Source: CAD feature listing. Evaluate the final solid. Frame: model axes, mm. A direction names the side the tool comes from. Give positions to 0.01 mm unless a question says otherwise; leave off trailing zeros. Loops run counter-clockwise (first coordinate to the right, second up) from the corner with the lowest first, then second, coordinate; pieces in that order, holes last.
```python
from build123d import *

# Parameters (mm, degrees)
SKETCH_1_W          = 16.2
SKETCH_1_H          = 16.9
EXTRUDE_1_DEPTH     = 16.9
CUT_EXTRUDE_1_DEPTH = 10
SKETCH_3_W          = 2.946300562
SKETCH_3_H          = 2.060350043
CUT_EXTRUDE_2_DEPTH = 0.2
SKETCH_4_W          = 14.323300114
SKETCH_4_H          = 2.725353119
CUT_EXTRUDE_3_DEPTH = 0.1
SKETCH_5_W          = 12.529891582
SKETCH_5_H          = 0.500524342
CUT_EXTRUDE_4_DEPTH = 0.1
CHAMFER_1_SIZE      = 0.5
CUT_EXTRUDE_5_DEPTH = 0.1
FILLET_1_R          = 0.1
SKETCH_7_R          = 1.25
SKETCH_7_W          = 0.5
SKETCH_7_H          = 0.4
SKETCH_7_H_2        = 0.5
SKETCH_7_W_2        = 0.3
SKETCH_7_H_3        = 1.2
EXTRUDE_2_DEPTH     = 3.3


with BuildPart() as part:
    # Эскиз1 → Бобышка-Вытянуть1 (new body)
    with BuildSketch(Plane.XY):
        Rectangle(SKETCH_1_W, SKETCH_1_H)
    extrude(amount=EXTRUDE_1_DEPTH)

    # Эскиз2 → Вырез-Вытянуть1 (cut)
    with BuildSketch(Plane.XY.offset(16.9)):
        Polygon((-6.264945791, -3.803921673), (-6.264945791, 4.664369649), (-3.10783524, 4.664369649), (-3.10783524, 6.730894781), (-1.828998264, 6.730894781), (-1.828998264, 7.89024711), (1.828998264, 7.89024711), (1.828998264, 6.730894781), (3.10783524, 6.730894781), (3.10783524, 4.664369649), (6.264945791, 4.664369649), (6.264945791, -3.803921673), align=None)
    extrude(amount=-CUT_EXTRUDE_1_DEPTH, mode=Mode.SUBTRACT)

    # Эскиз3 → Вырез-Вытянуть2 (cut)
    with BuildSketch(Plane.XY.offset(16.9)):
        with Locations((-5.415203287, 6.790232272)):
            Rectangle(SKETCH_3_W, SKETCH_3_H)
        with Locations((5.415203287, 6.790232272)):
            Rectangle(SKETCH_3_W, SKETCH_3_H)
    extrude(amount=-CUT_EXTRUDE_2_DEPTH, mode=Mode.SUBTRACT)

    # Эскиз4 → Вырез-Вытянуть3 (cut)
    with BuildSketch(Plane.XY.offset(16.9)):
        with Locations((0, 6.527570551)):
            Rectangle(SKETCH_4_W, SKETCH_4_H)
    extrude(amount=-CUT_EXTRUDE_3_DEPTH, mode=Mode.SUBTRACT)

    # Эскиз5 → Вырез-Вытянуть4 (cut)
    with BuildSketch(Plane.XY.offset(16.9)):
        with Locations((0, 4.91463182)):
            Rectangle(SKETCH_5_W, SKETCH_5_H)
    extrude(amount=-CUT_EXTRUDE_4_DEPTH, mode=Mode.SUBTRACT)

    # Фаска1
    chamfer_1_edges = [part.edges().sort_by_distance(p)[0] for p in [
        (0, -3.803921673, 6.9),
        (-6.264945791, 0.430223988, 6.9),
        (-4.686390516, 4.664369649, 6.9),
        (-3.10783524, 5.697632215, 6.9),
        (-2.468416752, 6.730894781, 6.9),
        (-1.828998264, 7.310570945, 6.9),
        (0, 7.89024711, 6.9),
        (1.828998264, 7.310570945, 6.9),
        (2.468416752, 6.730894781, 6.9),
        (3.10783524, 5.697632215, 6.9),
        (4.686390516, 4.664369649, 6.9),
        (6.264945791, 0.430223988, 6.9),
    ]]
    chamfer(chamfer_1_edges, length=CHAMFER_1_SIZE)

    # Эскиз6 → Вырез-Вытянуть5 (cut)
    with BuildSketch(Plane.ZY.offset(8.1)):
        Polygon((16.758546947, 8.45), (13.561955432, 5.115115471), (13.561955432, -5.115115471), (16.758546947, -8.45), (16.9, -8.45), (16.9, -8.308546947), (13.766132229, -5.039099757), (13.766132229, 5.039099757), (16.9, 8.308546947), (16.9, 8.45), align=None)
    cut_extrude_5 = extrude(amount=-CUT_EXTRUDE_5_DEPTH, mode=Mode.SUBTRACT)

    # Зеркальное отражение1: Вырез-Вытянуть5 across plane
    add(cut_extrude_5.mirror(Plane(origin=(0, 0, 0), x_dir=(0, 0, 1), z_dir=(1, 0, 0))), mode=Mode.SUBTRACT)

    # Скругление1
    fillet_1_edges = [part.edges().sort_by_distance(p)[0] for p in [
        (-8.05, 8.45, 16.758546947),
        (-8.05, 8.308546947, 16.9),
        (-8.05, -8.308546947, 16.9),
        (-8.05, -8.45, 16.758546947),
        (8.05, 8.45, 16.758546947),
        (8.05, -8.45, 16.758546947),
        (8.05, -8.308546947, 16.9),
        (8.05, 8.308546947, 16.9),
    ]]
    fillet(fillet_1_edges, radius=FILLET_1_R)

    # Эскиз7 → Бобышка-Вытянуть2 (add)
    with BuildSketch(Plane(origin=(0, 0, 0), x_dir=(-1, 0, 0), z_dir=(0, 0, -1))):
        with Locations((-5.715, 1.72)):
            Circle(SKETCH_7_R)
        with Locations((5.715, 1.72)):
            Circle(SKETCH_7_R)
        with Locations((-4.492372984, -4.63)):
            Rectangle(SKETCH_7_W, SKETCH_7_H)
        with Locations((-3.222372984, -7.17)):
            Rectangle(SKETCH_7_W, SKETCH_7_H)
        with Locations((-1.952372984, -4.63)):
            Rectangle(SKETCH_7_W, SKETCH_7_H)
        with Locations((-0.682372984, -7.17)):
            Rectangle(SKETCH_7_W, SKETCH_7_H)
        with Locations((0.587627016, -4.63)):
            Rectangle(SKETCH_7_W, SKETCH_7_H)
        with Locations((1.857627016, -7.17)):
            Rectangle(SKETCH_7_W, SKETCH_7_H)
        with Locations((3.127627016, -4.63)):
            Rectangle(SKETCH_7_W, SKETCH_7_H)
        with Locations((4.397627016, -7.17)):
            Rectangle(SKETCH_7_W, SKETCH_7_H)
        with Locations((-6.325, 5.83)):
            Rectangle(SKETCH_7_W, SKETCH_7_H_2)
        with Locations((-3.785, 5.83)):
            Rectangle(SKETCH_7_W, SKETCH_7_H_2)
        with Locations((3.785, 5.83)):
            Rectangle(SKETCH_7_W, SKETCH_7_H_2)
        with Locations((6.325, 5.83)):
            Rectangle(SKETCH_7_W, SKETCH_7_H_2)
        with Locations((-7.95, -2.18)):
            Rectangle(SKETCH_7_W_2, SKETCH_7_H_3)
        with Locations((7.95, -2.18)):
            Rectangle(SKETCH_7_W_2, SKETCH_7_H_3)
    extrude(amount=EXTRUDE_2_DEPTH)


solid = part.part
```
(1) First-contact query: pin 1 (1.6 mm diameter, centred on x = -4, y = 7, fed in from +Z); pin 2 (3 mm diameter, centred on x = -5.5, z = -1, fed in from -Y); pin 3 (2 mm diameter, centred on x = 6, y = -1, fed in from -Z); pin 4 (0.6 mm diameter, centred on x = 4.5, z = -2, fed in from +Y). Flat tips, straight axial feed; report the tip coordinate or a pass-through.
A:
pin 1: stops at z = 16.8
pin 2: stops at y = -8.45
pin 3: stops at z = 0
pin 4: stops at y = 2.57
(2) Reachability of faces 1 (the flat face through (-2, 6.731, 12)), 2 (the flat face through (8.1, 0, 15)), 3 (the cylindrical face through (5.99, 0.5, -1.63)), 4 (the flat face through (6, 2, -3.3)), 5 (the flat face through (7.8, -2, -2)) from +Z, -Z, +X, -X, +Y, -Y: full face, straight path, thin tool, end or side. Return the list, or none.
A:
face 1: +Z
face 2: +Z, -Z, +X, +Y, -Y
face 3: -Z
face 4: -Z, +X, -X, +Y, -Y
face 5: -Z, +Y, -Y
(3) Section D-D, the plane y = -6.5. Return the cut outline in (x, z).
A:
outline: (-8.1, 0) - (8.1, 0) - (8.1, 14.89) - (8, 14.89) - (8, 15.17) - (8.1, 15.17) - (8.1, 16.9) - (-8.1, 16.9) - (-8.1, 15.17) - (-8, 15.17) - (-8, 14.89) - (-8.1, 14.89) - close
(4) Section A-A, the plane y = 1.72. Return the cut outline in (x, z) (3 decimals), then the cut area to 3 significant figures.
A:
outline: (-8.1, 0) - (-6.965, 0) - (-6.965, -3.3) - (-4.465, -3.3) - (-4.465, 0) - (4.465, 0) - (4.465, -3.3) - (6.965, -3.3) - (6.965, 0) - (8.1, 0) - (8.1, 13.562) - (8, 13.562) - (8, 13.766) - (8.1, 13.766) - (8.1, 16.9) - (6.265, 16.9) - (6.265, 7.4) - (5.765, 6.9) - (-5.765, 6.9) - (-6.265, 7.4) - (-6.265, 16.9) - (-8.1, 16.9) - (-8.1, 13.766) - (-8, 13.766) - (-8, 13.562) - (-8.1, 13.562) - close
area: 165 mm2
(5) Mould query, pull axis Y, two halves, no side actions, for faces 6 (the flat face through (0, 7.89, 13)), 7 (the flat face through (-6, 2, -3.3)). Classes: pulls with the +Y half, pulls with the -Y half, needs draft (parallel to the pull), parting line crosses it, or undercut.
A:
face 6: undercut
face 7: needs draft
(6) Section C-C, the plane y = 3.5. Return the cut outline in (x, z), then the cut area to 3 significant figures.
A:
outline: (-8.1, 0) - (8.1, 0) - (8.1, 13.56) - (8, 13.56) - (8, 13.77) - (8.1, 13.77) - (8.1, 16.9) - (6.26, 16.9) - (6.26, 7.4) - (5.76, 6.9) - (-5.76, 6.9) - (-6.26, 7.4) - (-6.26, 16.9) - (-8.1, 16.9) - (-8.1, 13.77) - (-8, 13.77) - (-8, 13.56) - (-8.1, 13.56) - close
area: 149 mm2
(7) Ray query, line 1 along X through (y, z) = (0.75, 15.5); line 2 along Y through (x, z) = (-1, 13.5); line 3 along Y through (x, z) = (5.75, 13.75). Return the intervals inside material, ascending.
A:
line 1: x = -8.1 to -6.26, 6.26 to 8.1
line 2: y = -8.45 to -3.8, 7.89 to 8.45
line 3: y = -8.45 to -3.8, 4.66 to 8.45
(8) Section B-B, the plane z = -1.75. Count the separate pieces of the cut face and the enclosed holes in it, then the cut area to 3 significant figures.
A:
separate pieces: 16
enclosed holes: 0
area: 13.1 mm2
